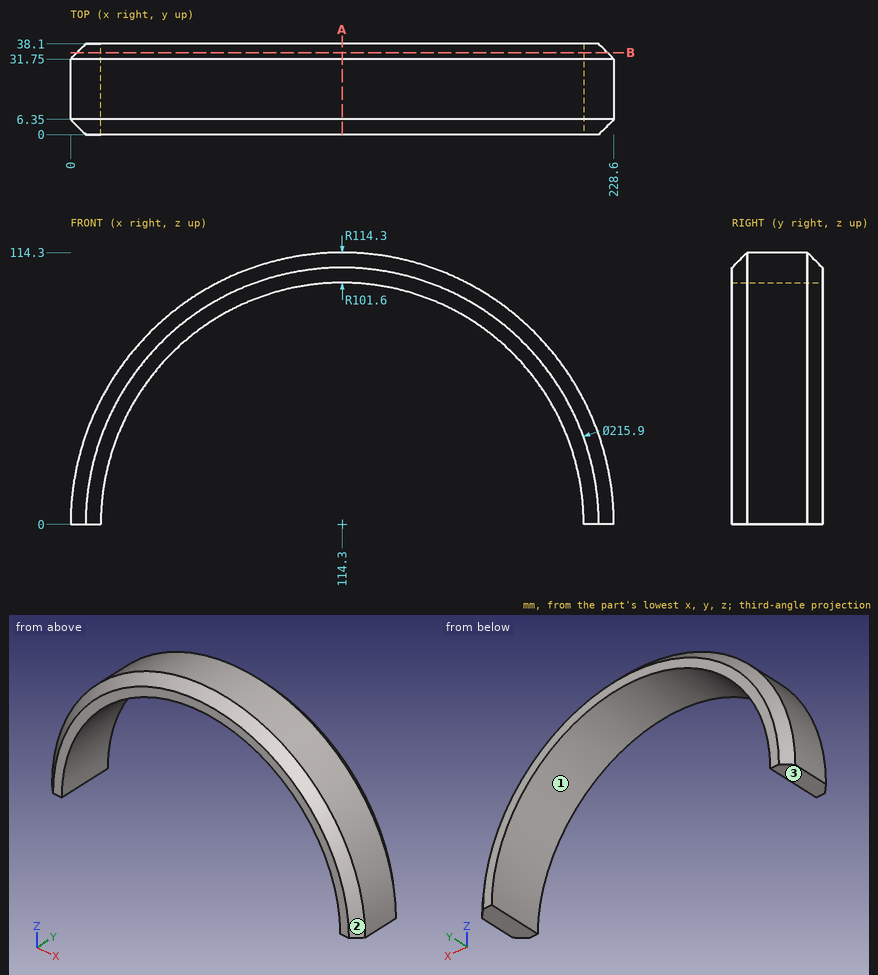
Input: dimensioned drawing with shaded views. Units: mm. Origin: part minimum x, y, z. Coordinates: 2 decimals unless noted, no trailing zeros. Loops run counter-clockwise (first coordinate to the right, second up) from the corner with the lowest first, then second, coordinate; pieces in that order, holes last. Notation, with made-up numbers: M -13,-6.75 L 43,-6.75 A17 ccw 43,5.25 Z; hole C 23,8.25 d6. An arc over 180 degrees is marked long. One line per item, written item: value.
(1) Pull-direction query (X, two-part tool) for the marked faces 1, 2 and 3; classes: +X half, -X half, draft (parallel to the pull), parting line (faces both ways), or undercut.
Filled in:
face 1: undercut
face 2: parting line
face 3: draft
(2) Line query: line 1 along X through (y, z) = (18, 51.5); line 2 along X through (y, z) = (26.5, 5); line 3 along Z through (x, y) = (85, 32.5). Output: solid intervals per line, ascending. Write a range as from..to.
Filled in:
line 1: 12.26..26.72, 201.88..216.34
line 2: 0.11..12.82, 215.78..228.49
line 3: 97.28..109.7
(3) Pin query (flat end, axial travel): pin 1 (2 mm diameter, centred on x = 192, y = 16.5, fed in from +Z); pin 2 (10 mm diameter, centred on y = 32.5, z = 38.5, fed in from +X); pin 3 (3 mm diameter, centred on x = 26.5, y = 33, fed in from +Z). Return the tip coordinate at first contact, or that it passes through.
Filled in:
pin 1: z = 84.74
pin 2: x = 223.56
pin 3: z = 74.17
(4) Section A-A (x = 114.3). Output: boundary loops of the cut face in (y, z), and give its area (3 significant figures).
Filled in:
outline: M 0,101.6 L 38.1,101.6 L 38.1,107.95 L 31.75,114.3 L 6.35,114.3 L 0,107.95 Z
area: 444 mm^2
(5) Section B-B (y = 34.5). Output: boundary loops of the cut face in (x, z).
Filled in:
outline: M 2.75,0 L 12.7,0 A101.6 cw 215.9,0 L 225.85,0 A111.55 ccw Z
